Can you work these out from the model? Positions are in its coordinate system, mm. A direction names the side the tool comes from. Give positions to 0.01 mm unless a question says otherwise; leave off trailing zeros. Loops run counter-clockwise (first coordinate to the right, second up) from the corner with the lowest first, then second, coordinate; pieces in that order, holes last. Notation, with made-up numbers: (-33.5, 35) - (-12.5, 35) arc R29 ccw to (-12.5, 56) - close; hole circle Ø11 at (51, 24.25). An arc over 180 degrees is marked (long way). Answer in a Markdown table with one row per item.
from build123d import *

# Parameters (mm, degrees)
SKETCH2_R                       = 48.5
SKETCH2_R_2                     = 1.5000000000000002
BOSS_EXTRUDE1_DEPTH             = 4
SKETCH3_R                       = 3.75
CUT_EXTRUDE1_DEPTH              = 1.5
BOSS_EXTRUDE3_START             = 4
SKETCH5_R                       = 9
BOSS_EXTRUDE3_DEPTH             = 14
CUT_EXTRUDE2_START              = 6
SKETCH9_R                       = 1.299999999999999
SKETCH9_R_2                     = 1.3000000000000043
SKETCH9_R_3                     = 1.2999999999999887
CUT_EXTRUDE2_DEPTH              = 96.33374378554642
BOSS_EXTRUDE6_DEPTH             = 9
BOSS_EXTRUDE6_DIRECTION_2_REACH = 113.079
CUT_EXTRUDE3_DEPTH              = 107.62868758356173
CUT_EXTRUDE3_DEPTH_BACK         = 107.62868758356173
FILLET2_R                       = 10
FILLET3_R                       = 2
FILLET4_R                       = 2


# Some blends are built 0.0001 mm under size
with BuildPart() as part:
    # Sketch2 → Boss-Extrude1 (new body)
    with BuildSketch(Plane(origin=(0, 0, 0), x_dir=(1, 0, 0), z_dir=(0, 1, 0))):
        with Locations(Location((0, 0, 0), (0, 0, 270))):
            Circle(SKETCH2_R)
        with Locations(Location((-2.66e-15, 7.249999999999999, 0), (0, 0, 270))):
            Circle(SKETCH2_R_2, mode=Mode.SUBTRACT)
        with Locations(Location((0, -7.249999999999999, 0), (0, 0, 270))):
            Circle(SKETCH2_R_2, mode=Mode.SUBTRACT)
    extrude(amount=BOSS_EXTRUDE1_DEPTH)

    # Sketch3 → Cut-Extrude1 (cut)
    with BuildSketch(Plane.XZ):
        with Locations(Location((0, 0, 0), (0, 0, 270))):
            Circle(SKETCH3_R)
    extrude(amount=-CUT_EXTRUDE1_DEPTH, mode=Mode.SUBTRACT)

    # Sketch5 → Boss-Extrude3 (add)
    with BuildSketch(Plane(origin=(0, 0, 0), x_dir=(0, 0, -1), z_dir=(1, 0, 0)).offset(BOSS_EXTRUDE3_START)):
        with BuildLine():
            Line((30.34, 4), (-30.34, 4))
            Line((-30.34, 4), (-30.34, 11.860000000000001))
            ThreePointArc((-30.34, 11.860000000000001), (-29.57328688616134, 19.16990813910404), (-27.306519613843914, 26.161644127699585))
            Line((-27.306519613843914, 26.161644127699585), (-13.792358873261465, 56.585344889913266))
            ThreePointArc((-13.792358873261465, 56.585344889913266), (31.303559206891457, 69.10551707656947), (34.93556554151654, 22.444986978202348))
            ThreePointArc((34.93556554151654, 22.444986978202348), (31.53662148462827, 17.510838233282712), (30.34, 11.64))
            Line((30.34, 11.64), (30.34, 4))
        make_face()
        with Locations((13.909999999999995, 44.28)):
            Circle(SKETCH5_R, mode=Mode.SUBTRACT)
    extrude(amount=BOSS_EXTRUDE3_DEPTH)

    # Sketch9 → Cut-Extrude2 (cut, through all)
    with BuildSketch(Plane(origin=(0, 0, 0), x_dir=(0, 0, -1), z_dir=(1, 0, 0)).offset(CUT_EXTRUDE2_START)):
        with Locations(Location((29.540705350702062, 50.78483624530012, 0), (0, 0, 180))):
            Circle(SKETCH9_R)
        with Locations(Location((22.87605932116741, 58.24020299020328, 0), (0, 0, 180))):
            Circle(SKETCH9_R)
        with Locations(Location((-7.795885678067851, 17.4081866892785, 0), (0, 0, 180))):
            Circle(SKETCH9_R_2)
        with Locations(Location((-14.460531707602502, 24.86355343418166, 0), (0, 0, 180))):
            Circle(SKETCH9_R_3)
        Polygon((0, 17), (29.075930305122334, 42.99211951518514), (15.080173643099549, 58.648389679481774), (-13.99575666202277, 32.65627016429665), align=None)
    extrude(amount=CUT_EXTRUDE2_DEPTH, mode=Mode.SUBTRACT)

    # Sketch11 → Boss-Extrude6 (add)
    with BuildSketch(Plane(origin=(18.000000000000004, 0, 0), x_dir=(0, 0, -1), z_dir=(1, 0, 0))):
        with BuildLine():
            ThreePointArc((39.09733932490991, 18.12299218692141), (34.7464182617029, 74.01944844856713), (-19.27572866273243, 59.02104925455133))
            Line((-19.27572866273244, 59.021049254551315), (-32.78988940331492, 28.59734849233759))
            ThreePointArc((-32.78988940331492, 28.59734849233759), (-35.44270843929697, 20.41485417471641), (-36.34, 11.860000000000007))
            Line((-36.34, 11.860000000000007), (-36.34, 4))
            Line((-36.34, 4), (-30.34, 4.000000000000001))
            Line((-30.34, 4), (-30.34, 11.860000000000001))
            ThreePointArc((-30.339999999999996, 11.860000000000003), (-29.573286886161334, 19.169908139104034), (-27.30651961384391, 26.161644127699585))
            Line((-27.30651961384391, 26.161644127699585), (-19.28989223747492, 44.20904471014288))
            ThreePointArc((-19.289892237474774, 44.20904471014282), (-16.709962361716535, 50.472191847815), (-13.792358873261435, 56.58534488991329))
            ThreePointArc((-13.79235887326144, 56.58534488991327), (31.303559206891478, 69.10551707656947), (34.935565541516546, 22.444986978202333))
            ThreePointArc((34.93556554151654, 22.444986978202337), (31.536621484628263, 17.510838233282712), (30.339999999999996, 11.64))
            Line((30.34, 11.64), (30.34, 4))
            Line((30.34, 4), (36.34, 4))
            Line((36.34, 4), (36.34, 11.64))
            ThreePointArc((36.34, 11.64), (37.05797289077695, 15.162502939969631), (39.09733932490992, 18.122992186921408))
        make_face()
    extrude(amount=BOSS_EXTRUDE6_DEPTH)

    # Boss-Extrude6 direction 2: up to this face of the body (flat: up to its plane)
    boss_extrude6_direction_2_end = Plane(part.part.faces().sort_by_distance((4, 35.761181815, -7.797700276))[0])
    # Sketch11 → Boss-Extrude6 direction 2 (add, up to the picked face)
    with BuildSketch(Plane(origin=(18.000000000000004, 0, 0), x_dir=(0, 0, -1), z_dir=(1, 0, 0)), mode=Mode.PRIVATE) as boss_extrude6_direction_2_sk1:
        with BuildLine():
            ThreePointArc((39.09733932490991, 18.12299218692141), (34.7464182617029, 74.01944844856713), (-19.27572866273243, 59.02104925455133))
            Line((-19.27572866273244, 59.021049254551315), (-32.78988940331492, 28.59734849233759))
            ThreePointArc((-32.78988940331492, 28.59734849233759), (-35.44270843929697, 20.41485417471641), (-36.34, 11.860000000000007))
            Line((-36.34, 11.860000000000007), (-36.34, 4))
            Line((-36.34, 4), (-30.34, 4.000000000000001))
            Line((-30.34, 4), (-30.34, 11.860000000000001))
            ThreePointArc((-30.339999999999996, 11.860000000000003), (-29.573286886161334, 19.169908139104034), (-27.30651961384391, 26.161644127699585))
            Line((-27.30651961384391, 26.161644127699585), (-19.28989223747492, 44.20904471014288))
            ThreePointArc((-19.289892237474774, 44.20904471014282), (-16.709962361716535, 50.472191847815), (-13.792358873261435, 56.58534488991329))
            ThreePointArc((-13.79235887326144, 56.58534488991327), (31.303559206891478, 69.10551707656947), (34.935565541516546, 22.444986978202333))
            ThreePointArc((34.93556554151654, 22.444986978202337), (31.536621484628263, 17.510838233282712), (30.339999999999996, 11.64))
            Line((30.34, 11.64), (30.34, 4))
            Line((30.34, 4), (36.34, 4))
            Line((36.34, 4), (36.34, 11.64))
            ThreePointArc((36.34, 11.64), (37.05797289077695, 15.162502939969631), (39.09733932490992, 18.122992186921408))
        make_face()
    boss_extrude6_direction_2_tool1 = split(extrude(boss_extrude6_direction_2_sk1.sketch, amount=-BOSS_EXTRUDE6_DIRECTION_2_REACH, mode=Mode.PRIVATE), bisect_by=boss_extrude6_direction_2_end, keep=Keep.BOTH, mode=Mode.PRIVATE)
    add(boss_extrude6_direction_2_tool1.solids().sort_by(Axis((18, 73.072836, -34.083191), (-1, 0, 0)))[0])

    # Sketch14 → Cut-Extrude3 (cut, two sides: drawn at the far end of the back side and taken through both)
    with BuildSketch(Plane.XY.offset(-CUT_EXTRUDE3_DEPTH_BACK)):
        with BuildLine():
            Line((27.00000000000001, 80.59240999991061), (21.00000000000001, 80.59240999991061))
            ThreePointArc((21.00000000000001, 80.59240999991061), (25.222549691509585, 42.401946852226466), (26.500000000000004, 4))
            Line((26.500000000000004, 4), (27.000000000000004, 4))
            Line((27.000000000000004, 4), (27.00000000000001, 80.59240999991061))
        make_face()
    extrude(amount=CUT_EXTRUDE3_DEPTH + CUT_EXTRUDE3_DEPTH_BACK, mode=Mode.SUBTRACT)

    # Fillet2
    # the kernel refuses this fillet: 10 mm, written as the material it takes off along each edge
    with BuildSketch(Plane(origin=(4, 11.860000000000007, 36.34), x_dir=(0, 0, -1), z_dir=(0, -1, 0))) as fillet2_piece_1:
        with BuildLine():
            CenterArc((FILLET2_R, FILLET2_R), FILLET2_R, 180, 90)
            Line((0, FILLET2_R), (0, 0))
            Line((0, 0), (FILLET2_R, 0))
        make_face()
    extrude(amount=7.8600000000000065, mode=Mode.SUBTRACT)
    with BuildSketch(Plane(origin=(4, 11.86, -4.889999999999912), x_dir=(0, 0.4059507274396709, 0.9138949649118339), z_dir=(0, 0.9138949649118339, -0.4059507274396709))) as fillet2_piece_2:
        with BuildLine():
            CenterArc((41.22999999999991 - FILLET2_R, FILLET2_R), FILLET2_R, 270, 89.99999999999999)
            Line((41.22999999999991, FILLET2_R), (41.22999999999991, 0))
            Line((41.22999999999991, 0), (41.22999999999991 - FILLET2_R, 0))
        make_face()
    revolve(axis=Axis((4, 11.86, -4.889999999999912), (1, 0, 0)), revolution_arc=23.950718342801608, mode=Mode.SUBTRACT)
    with BuildSketch(Plane(origin=(4, 59.02104925455132, 19.275728662732437), x_dir=(0, -0.4059507274396704, -0.9138949649118341), z_dir=(0, -0.9138949649118341, 0.40595072743967037))) as fillet2_piece_3:
        with BuildLine():
            CenterArc((FILLET2_R, FILLET2_R), FILLET2_R, 180, 90)
            Line((-3.25e-15, FILLET2_R), (0, 0))
            Line((0, 0), (FILLET2_R, 0))
        make_face()
    extrude(amount=33.29015032394755, mode=Mode.SUBTRACT)
    with BuildSketch(Plane(origin=(4, 44.28, -13.909999999999988), x_dir=(0, -0.7203324652134898, -0.6936289638988963), z_dir=(0, -0.6936289638988963, 0.7203324652134898))) as fillet2_piece_4:
        with BuildLine():
            CenterArc((36.312409999910614 - FILLET2_R, FILLET2_R), FILLET2_R, 270, 89.99999999999999)
            Line((36.312409999910614, FILLET2_R), (36.312409999910614, 0))
            Line((36.312409999910614, 0), (36.312409999910614 - FILLET2_R, 0))
        make_face()
    revolve(axis=Axis((4, 44.28, -13.909999999999988), (1, 0, 0)), revolution_arc=202.13121786262028, mode=Mode.SUBTRACT)
    with BuildSketch(Plane(origin=(4, 4, -36.34), x_dir=(0, 0, 1), z_dir=(0, 1, 0))) as fillet2_piece_5:
        with BuildLine():
            CenterArc((FILLET2_R, FILLET2_R), FILLET2_R, 180, 90)
            Line((0, FILLET2_R), (0, 0))
            Line((0, 0), (FILLET2_R, 0))
        make_face()
    extrude(amount=7.640000000000001, mode=Mode.SUBTRACT)
    with BuildSketch(Plane(origin=(4, 11.640000000000043, -45.33999999999995), x_dir=(0, 0.7203324652134898, 0.6936289638988964), z_dir=(0, 0.6936289638988964, -0.7203324652134898))) as fillet2_piece_6:
        with BuildLine():
            CenterArc((8.999999999999945 + FILLET2_R, FILLET2_R), FILLET2_R, 180, 90)
            Line((8.999999999999941, FILLET2_R), (8.999999999999945, 0))
            Line((8.999999999999945, 0), (8.999999999999945 + FILLET2_R, 0))
        make_face()
    revolve(axis=Axis((4, 11.640000000000043, -45.33999999999995), (1, 0, 0)), revolution_arc=46.08193620542221, mode=Mode.SUBTRACT)

    # Fillet3
    fillet3_edges = [part.edges().sort_by_distance(p)[0] for p in [
        (20.250000000000014, 4, -36.34),
        (4, 4, 0),
        (20.250000000000014, 4, 36.34),
        (6.928932188134525, 4, -33.41106781186548),
        (6.928932188134525, 3.999999999999999, 33.41106781186548),
    ]]
    fillet(fillet3_edges, radius=FILLET3_R)

    # Fillet4
    fillet4_edges = [part.edges().sort_by_distance(p)[0] for p in [
        (26.500000000000032, 4.000000000000001, -34.34),
        (26.500000000000036, 4.000000000000001, 34.34),
    ]]
    fillet(fillet4_edges, radius=FILLET4_R - 0.0001)  # a hair under: the kernel refuses the full size


solid = part.part
Q1. On a 3-axis mill with a long thin cutter (end or side, diameter ignored), from which of +Z, -Z, +X, -X, +Y, -Y can I reach the whole of each face in a straight line? I mean faces 4 (the face through (0.165, 0.74, 3.746)), 5 (the face through (20, 9, 36.34)), 6 (the face through (11.916, 50.711, -22.176)). Say none if no direction works.
Checked values:
| item | result |
|---|---|
| face 4 | -Y |
| face 5 | +Z, +X, -X, +Y |
| face 6 | +X |
Q2. Imagine slicing it at A-A, the plane y = 7.5. Write out the boundary of the cut face in (x, z), and give its area (3 significant figures).
Checked values:
| item | result |
|---|---|
| outline | (4, -26.34) arc R10 ccw to (14, -36.34) - (26.51, -36.34) - (26.51, -30.34) - (18, -30.34) - (18, 30.34) - (26.51, 30.34) - (26.51, 36.34) - (14, 36.34) arc R10 ccw to (4, 26.34) - close |
| area | 1,080 mm² |
Q3. Imagine slicing it at C-C, the plane x = -38. Write out the boundary of the cut face in (y, z), and give its area (3 significant figures).
Checked values:
| item | result |
|---|---|
| outline | (0, -30.14) - (4, -30.14) - (4, 30.14) - (0, 30.14) - close |
| area | 241 mm² |
Q4. If we mould it in two halves opening along Z, with no side actions, what happens to faces 1 (the face through (21.15, 61.2, -39.06)), 2 (the face through (-43.028, 1.972, 22.38)), 3 (the face through (7.01, 8.78, -33.49))? For each: released by +Z, released by -Z, zero draft, split by the parting line, or undercut.
Checked values:
| item | result |
|---|---|
| face 1 | undercut |
| face 2 | split by the parting line |
| face 3 | released by -Z |
Q5. If I drill on line 1 (X direction, y = 0.6, z = 0); line 2 (Y direction, x = 33, z = 14); line 3 (X direction, y = 46.5, z = -32.5), over which ranges is the centre line in solid material (lowest first)? Write a range as [from, to].
Checked values:
| item | result |
|---|---|
| line 1 | x = [-48.5, -3.75], [3.75, 48.5] |
| line 2 | y = [0, 4] |
| line 3 | x = [4, 18] |
Q6. For pin 1 (4 mm diameter, centred on x = 0, z = 7.25, fed in from +Y); pin 2 (12 mm diameter, centred on x = 0, z = 0, fed in from +Y); pin 3 (0.8 mm diameter, centred on y = 17.5, z = 8, fed in from +X); pin 4 (1.5 mm diameter, centred on x = 28.5, y = 10, fed in from -Z), each with a flat end and sliding along its axis, tell me the tip position at first contact or that it passes through.
Checked values:
| item | result |
|---|---|
| pin 1 | stops at y = 4 |
| pin 2 | stops at y = 73.83 |
| pin 3 | stops at x = 6 |
| pin 4 | passes through |
Q7. Imagine slicing it at B-B, the plane z = -7.25. Count the separate pieces of the cut face and the enclosed holes in it, and give its area (3 significant figures).
Checked values:
| item | result |
|---|---|
| separate pieces | 3 |
| enclosed holes | 0 |
| area | 1,070 mm² |
